from build123d import *

# Parameters (mm, degrees)
SKETCH1_W           = 28
SKETCH1_H           = 40
BOSS_EXTRUDE1_DEPTH = 3
SKETCH2_R           = 14
BOSS_EXTRUDE2_DEPTH = 7
SKETCH3_R           = 8.5
BOSS_EXTRUDE3_DEPTH = 2
FILLET1_R           = 1
SKETCH4_R           = 0.884555984
SKETCH4_R_2         = 0.79363575
BOSS_EXTRUDE4_DEPTH = 8
SKETCH5_W           = 5.850646162
SKETCH5_H           = 7.111200286
BOSS_EXTRUDE5_DEPTH = 5
SKETCH6_R           = 1.5
CUT_EXTRUDE1_DEPTH  = 5
CUT_EXTRUDE2_DEPTH  = 1.5
CUT_EXTRUDE2_DRAFT  = -30
SKETCH8_R           = 6.5
BOSS_EXTRUDE6_DEPTH = 1
FILLET2_R           = 1


with BuildPart() as part:
    # Sketch1 → Boss-Extrude1 (new body)
    with BuildSketch(Plane.XY):
        Rectangle(SKETCH1_W, SKETCH1_H)
    extrude(amount=BOSS_EXTRUDE1_DEPTH)

    # Sketch2 → Boss-Extrude2 (add)
    with BuildSketch(Plane.XY.offset(3)):
        Circle(SKETCH2_R)
    extrude(amount=BOSS_EXTRUDE2_DEPTH)

    # Sketch3 → Boss-Extrude3 (add)
    with BuildSketch(Plane.XY.offset(10)):
        Circle(SKETCH3_R)
    extrude(amount=BOSS_EXTRUDE3_DEPTH)

    # Fillet1
    fillet1_edges = [part.edges().sort_by_distance(p)[0] for p in [
        (-8.5, 0, 12),
    ]]
    fillet(fillet1_edges, radius=FILLET1_R)

    # Sketch4 → Boss-Extrude4 (add)
    with BuildSketch(Plane.XY.offset(3)):
        with BuildLine():
            ThreePointArc((-8.575515757, -17.151031514), (0, -19.175436175), (8.575515757, -17.151031514))
            ThreePointArc((8.575515757, -17.151031514), (9.469942948, -14.467749941), (6.786661375, -13.57332275))
            ThreePointArc((6.786661375, -13.57332275), (0, -15.175436175), (-6.786661375, -13.57332275))
            ThreePointArc((-6.786661375, -13.57332275), (-9.469942948, -14.467749941), (-8.575515757, -17.151031514))
        make_face()
        with Locations((7.681088566, -15.362177132)):
            Circle(SKETCH4_R, mode=Mode.SUBTRACT)
        with Locations((-7.681088566, -15.362177132)):
            Circle(SKETCH4_R_2, mode=Mode.SUBTRACT)
    extrude(amount=BOSS_EXTRUDE4_DEPTH)

    # Sketch5 → Boss-Extrude5 (add)
    with BuildSketch(Plane.XY.offset(3)):
        with Locations((0.05792719, 16.444399857)):
            Rectangle(SKETCH5_W, SKETCH5_H)
    extrude(amount=BOSS_EXTRUDE5_DEPTH)

    # Sketch6 → Cut-Extrude1 (cut)
    with BuildSketch(Plane.XY.offset(3)):
        with Locations((-11.5, 17)):
            Circle(SKETCH6_R)
        with Locations((11.5, 17)):
            Circle(SKETCH6_R)
        with Locations((11.5, -17)):
            Circle(SKETCH6_R)
        with Locations((-11.5, -17)):
            Circle(SKETCH6_R)
    extrude(amount=-CUT_EXTRUDE1_DEPTH, mode=Mode.SUBTRACT)


with BuildPart() as cut_extrude2_tool:
    # Sketch7 → Cut-Extrude2 (with draft: the straight prism first)
    with BuildSketch(Plane(origin=(0, 0, 0), x_dir=(-1, 0, 0), z_dir=(0, 0, -1))):
        with BuildLine():
            ThreePointArc((-12, -5), (0, -17), (12, -5))
            Line((12, -5), (12, 5))
            ThreePointArc((12, 5), (0, 17), (-12, 5))
            Line((-12, 5), (-12, -5))
        make_face()
    extrude(amount=-CUT_EXTRUDE2_DEPTH)
    # Cut-Extrude2: the draft: its side faces are tilted about the plane it starts from
    cut_extrude2_sides = [cut_extrude2_tool.faces().sort_by_distance(p)[0] for p in [
        (-12, 0, 0.75),
        (0, 17, 0.75),
        (12, 0, 0.75),
        (0, -17, 0.75),
    ]]
    draft(cut_extrude2_sides, Plane(origin=(0, 0, 0), x_dir=(-1, 0, 0), z_dir=(0, 0, -1)), CUT_EXTRUDE2_DRAFT)


with BuildPart() as part_1:
    add(part.part)

    # Cut-Extrude2: cut by cut_extrude2_tool
    add(cut_extrude2_tool.part, mode=Mode.SUBTRACT)

    # Sketch8 → Boss-Extrude6 (add)
    with BuildSketch(Plane(origin=(0, 0, 1.5), x_dir=(-1, 0, 0), z_dir=(0, 0, -1))):
        Circle(SKETCH8_R)
    extrude(amount=BOSS_EXTRUDE6_DEPTH)

    # Fillet2
    fillet2_edges = [part_1.edges().sort_by_distance(p)[0] for p in [
        (6.5, 0, 0.5),
    ]]
    fillet(fillet2_edges, radius=FILLET2_R - 0.0001)  # a hair under: the kernel refuses the full size


solid = part_1.part
The listing builds one solid part. Answer for the finished solid, in the listing's coordinates (mm). A direction names the side the tool comes from. Round coordinates to 2 decimals unless told otherwise and drop trailing zeros. Loops run counter-clockwise (first coordinate to the right, second up) from the corner with the lowest first, then second, coordinate; pieces in that order, holes last. Notation, with made-up numbers: M -38.75,53.25 L 18.25,53.25 A22 cw 18.25,71.25 Z; hole C -35.75,65.25 d9. An arc over 180 degrees is marked long. Return JSON: item names as keys, results as strings.
Q1. The mould has two halves that part along X. Classify faces 4 (the face through (8.089, -16.147, 6.944)), 5 (the face through (2.983, 17, 5)), 6 (the face through (-8, -15, 3)), 7 (the face through (0, 0, 12)): released by +X, released by -X, zero draft, split by the parting line, or undercut.
Results list:
{"face 4": "undercut", "face 5": "released by +X", "face 6": "undercut", "face 7": "zero draft"}
Q2. Find section B-B, the plane z = 6.5. Determine the outline of the cut face in (x, y).
Results list:
{"outline": "M -8.58,-17.15 A19.18 ccw 8.58,-17.15 A2 ccw 6.79,-13.57 A15.18 cw -6.79,-13.57 A2 ccw Z; M -2.87,13.7 A14 ccw long 2.98,13.68 L 2.98,20 L -2.87,20 Z; hole C -7.68,-15.36 d1.59; hole C 7.68,-15.36 d1.77"}
Q3. Find the intervals of material crossed by line 1 along Y through (x, z) = (11.5, 1.35); line 2 along Z through (x, y) = (5, -14.5); line 3 along Z through (x, y) = (7.5, -10), in increasing order. Write a range as from..to.
Results list:
{"line 1": "y = -20..-18.5, -15.5..15.5, 18.5..20", "line 2": "z = 1.5..11", "line 3": "z = 1.5..10"}
Q4. Which of the six approach directions +Z, -Z, +X, -X, +Y, -Y give full straight-line access (tool end or side, diameter ignored) to faces 1 (the face through (-10, 15, 3)), 2 (the face through (-0.25, 16.28, 1.24)), 3 (the face through (8, -15, 3))?
Results list:
{"face 1": "+Z, -X, +Y", "face 2": "-Z", "face 3": "+Z"}
Q5. Find section A-A, the plane z = 10.5. Determine the outline of the cut face in (x, y).
Results list:
{"outline": "M -8.58,-17.15 A19.18 ccw 8.58,-17.15 A2 ccw 6.79,-13.57 A15.18 cw -6.79,-13.57 A2 ccw Z; C 0,0 d17; hole C -7.68,-15.36 d1.59; hole C 7.68,-15.36 d1.77"}
Q6. Each of these flat-tipped pins is pushed along its axis until it touches: pin 1 Ø5.5 at (y, z) = (16.5, 6.5) entering from +X; pin 2 Ø4 at (y, z) = (-3.5, 3.5) entering from +X; pin 3 Ø3.5 at (x, y) = (1, 1.5) entering from -Z; pin 4 Ø2.5 at (x, y) = (-11.5, 17) entering from +Z. Where does it stop, or does it pass through?
Results list:
{"pin 1": "stops at x = 2.98", "pin 2": "stops at x = 14", "pin 3": "stops at z = 0.5", "pin 4": "passes through"}
Q7. Find section C-C, the plane z = 8.5. Determine the outline of the cut face in (x, y), plus the area to 3 significant figures.
Results list:
{"outline": "C 0,0 d28; M -8.58,-17.15 A19.18 ccw 8.58,-17.15 A2 ccw 6.79,-13.57 A15.18 cw -6.79,-13.57 A2 ccw Z; hole C -7.68,-15.36 d1.59; hole C 7.68,-15.36 d1.77", "area": "688 mm2"}
